Can you work these out from the model? Positions are in its coordinate system, mm. Face numbers are marked on the shaded views. Round coordinates to 2 decimals unless told otherwise and drop trailing zeros. Loops run counter-clockwise (first coordinate to the right, second up) from the corner with the lowest first, then second, coordinate; pieces in that order, holes last. Notation, with made-up numbers: M 14.5,83.5 L 63.5,83.5 A4 ccw 63.5,88.5 Z; hole C -18,69 d11. An arc over 180 degrees is marked long. Use a Markdown table: item, result. Add a question column.
```python
from build123d import *

# Parameters (mm, degrees)
SKETCH_1_W          = 21.66025404
SKETCH_1_H          = 40
EXTRUDE_1_DEPTH     = 5
CUT_EXTRUDE_1_DEPTH = 40
SKETCH_3_R          = 1.15
CUT_EXTRUDE_2_DEPTH = 5


with BuildPart() as part:
    # Эскиз1 → Бобышка-Вытянуть1 (new body)
    with BuildSketch(Plane(origin=(0, 0, 0), x_dir=(1, 0, 0), z_dir=(0, 1, 0))):
        Rectangle(SKETCH_1_W, SKETCH_1_H)
    extrude(amount=EXTRUDE_1_DEPTH)

    # Эскиз2 → Вырез-Вытянуть1 (cut)
    with BuildSketch(Plane.XY.offset(20)):
        with BuildLine():
            Line((-4.33012702, 0), (4.33012702, 0))
            ThreePointArc((4.33012702, 0), (0, 2.500000002), (-4.33012702, 0))
        make_face()
    extrude(amount=-CUT_EXTRUDE_1_DEPTH, mode=Mode.SUBTRACT)

    # Эскиз3 → Вырез-Вытянуть2 (cut)
    with BuildSketch(Plane.XZ):
        with Locations(Location((7.58012702, 12.5, 0), (0, 0, 270))):
            Circle(SKETCH_3_R)
        with Locations(Location((7.58012702, -12.5, 0), (0, 0, 270))):
            Circle(SKETCH_3_R)
        with Locations(Location((7.58012702, 0, 0), (0, 0, 270))):
            Circle(SKETCH_3_R)
        with Locations(Location((-7.58012702, -12.5, 0), (0, 0, 270))):
            Circle(SKETCH_3_R)
        with Locations(Location((-7.58012702, 0, 0), (0, 0, 270))):
            Circle(SKETCH_3_R)
        with Locations(Location((-7.58012702, 12.5, 0), (0, 0, 270))):
            Circle(SKETCH_3_R)
    extrude(amount=-CUT_EXTRUDE_2_DEPTH, mode=Mode.SUBTRACT)


solid = part.part
```
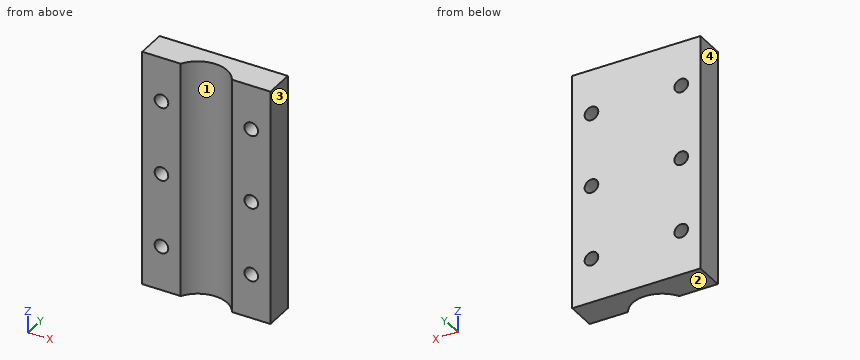
(1) Suppose I cut it at C-C on y = 4.45. List the corners of the cut face in (x, z) for me.
(2) If I drill on probe 1 along Z at (x, y) = (7.5, 1.5); probe 2 along X at (y, z) = (3.8, 12.5); probe 3 along X at (y, z) = (1.9, -12.5), over which ranges is the centre line in solid material (lowest first)? Write a range as [from, to].
(3) I'm going to push flat-ended pins straight in: pin 1 (3 mm diameter, centred on x = 7.58, z = 0, fed in from +Y); pin 2 (2 mm diameter, centred on x = 1.5, z = -13.5, fed in from -Y). Where does each tip first touch, or does it pass through?
(4) Suppose I cut it at A-A on y = 2. List the corners of the cut face in (x, z) for me, and give its area (3 significant figures).
(5) Suppose I cut it at D-D on x = -1. List the corners of the cut face in (y, z) for me.
(6) Suppose I cut it at B-B on z = 12.5. List the corners of the cut face in (x, y) for me, and give its area (3 significant figures).
(7) Thinking about a two-plate mould opening in X: for the marked faces 1, 2, 3 and 4, which applies, released by +X, released by -X, zero draft, split by the parting line, or undercut?
Results below:
| question | item | result |
|---|---|---|
| 1 | outline | M -10.83,-20 L 10.83,-20 L 10.83,20 L -10.83,20 Z; hole C -7.58,-12.5 d2.3; hole C -7.58,0 d2.3; hole C -7.58,12.5 d2.3; hole C 7.58,-12.5 d2.3; hole C 7.58,0 d2.3; hole C 7.58,12.5 d2.3 |
| 2 | probe 1 | z = [-20, -13.65], [-11.35, -1.15], [1.15, 11.35], [13.65, 20] |
| 2 | probe 2 | x = [-10.83, -8.73], [-6.43, 6.43], [8.73, 10.83] |
| 2 | probe 3 | x = [-10.83, -8.73], [-6.43, -2.37], [2.37, 6.43], [8.73, 10.83] |
| 3 | pin 1 | stops at y = 5 |
| 3 | pin 2 | stops at y = 1.83 |
| 4 | outline | M -10.83,-20 L -2.18,-20 L -2.18,20 L -10.83,20 Z; M 2.18,-20 L 10.83,-20 L 10.83,20 L 2.18,20 Z; hole C -7.58,-12.5 d2.3; hole C -7.58,0 d2.3; hole C -7.58,12.5 d2.3; hole C 7.58,-12.5 d2.3; hole C 7.58,0 d2.3; hole C 7.58,12.5 d2.3 |
| 4 | area | 667 mm² |
| 5 | outline | M 2.4,-20 L 5,-20 L 5,20 L 2.4,20 Z |
| 6 | outline | M -10.83,0 L -8.73,0 L -8.73,5 L -10.83,5 Z; M -6.43,0 L -4.33,0 A5 cw 4.33,0 L 6.43,0 L 6.43,5 L -6.43,5 Z; M 8.73,0 L 10.83,0 L 10.83,5 L 8.73,5 Z |
| 6 | area | 69.9 mm² |
| 7 | face 1 | undercut |
| 7 | face 2 | zero draft |
| 7 | face 3 | released by +X |
| 7 | face 4 | released by -X |
